from build123d import *

# Parameters (mm, degrees)
SKETCH_1_R               = 7.5
EXTRUDE_1_DEPTH          = 4
SKETCH_1_3_R             = 7.5
EXTRUDE_2_DEPTH          = 6
EXTRUDE_3_DEPTH          = 2
HOLE_WIZARD_M3_1_D       = 2.5
SKETCH_5_R               = 2.75
CUT_EXTRUDE_1_DEPTH      = 1
CUT_EXTRUDE_1_DEPTH_BACK = 4
SKETCH_6_R               = 4
CUT_EXTRUDE_2_DEPTH      = 0.75


with BuildPart() as part:
    # 草图1 → 凸台-拉伸1 (new body)
    with BuildSketch(Plane(origin=(0, 0, 0), x_dir=(1, 0, 0), z_dir=(0, 1, 0))):
        Circle(SKETCH_1_R)
        with BuildLine():
            Line((0, 3), (24.5, 3))
            ThreePointArc((24.5, 3), (27.5, 0), (24.5, -3))
            Line((24.5, -3), (0, -3))
            ThreePointArc((0, -3), (-3, 0), (0, 3))
        make_face()
    extrude(amount=EXTRUDE_1_DEPTH)

    # 草图1<3> → 凸台-拉伸2 (add)
    with BuildSketch(Plane(origin=(0, 0, 0), x_dir=(1, 0, 0), z_dir=(0, 1, 0))):
        Circle(SKETCH_1_3_R)
    extrude(amount=EXTRUDE_2_DEPTH)

    # 草图2 → 凸台-拉伸3 (add)
    with BuildSketch(Plane(origin=(0, 4, 0), x_dir=(1, 0, 0), z_dir=(0, 1, 0))):
        with BuildLine():
            Line((20, -2.5), (24, -2.5))
            ThreePointArc((24, -2.5), (26.5, 0), (24, 2.5))
            Line((24, 2.5), (20, 2.5))
            ThreePointArc((20, 2.5), (17.5, 0), (20, -2.5))
        make_face()
    extrude(amount=EXTRUDE_3_DEPTH)

    # M3 螺纹孔1 (through all)
    with Locations(Plane.XZ):
        with Locations((20, 0), (24, 0), (0, 0), (9, 0)):
            Hole(HOLE_WIZARD_M3_1_D / 2)

    # 草图5 → 切除-拉伸1 (cut, two sides)
    with BuildSketch(Plane(origin=(0, 6, 0), x_dir=(1, 0, 0), z_dir=(0, 1, 0))) as cut_extrude_1_sk:
        Circle(SKETCH_5_R)
    extrude(amount=CUT_EXTRUDE_1_DEPTH, mode=Mode.SUBTRACT)
    extrude(cut_extrude_1_sk.sketch, amount=-CUT_EXTRUDE_1_DEPTH_BACK, mode=Mode.SUBTRACT)

    # 草图6 → 切除-拉伸2 (cut)
    with BuildSketch(Plane.XZ):
        Circle(SKETCH_6_R)
    extrude(amount=-CUT_EXTRUDE_2_DEPTH, mode=Mode.SUBTRACT)


solid = part.part
Source: CAD feature listing. Evaluate the final solid. Frame: model axes, mm. A direction names the side the tool comes from. Give positions to 0.01 mm unless a question says otherwise; leave off trailing zeros. Write each loop counter-clockwise with the first axis right and the second up, starting at its lowest first coordinate (ties: lowest second). Pieces come first, ordered by that corner, then holes. Notation, with made-up numbers: (46, 25) -> (94, 25) arc R26 ccw to (94, 42) -> close; hole circle Ø1 at (68.5, 60.5). An arc over 180 degrees is marked (long way). Write item = value, one per line.
Q1. Mould query, pull axis X, two halves, no side actions, for faces 1 (the face through (-0.596, 4.028, 2.685)), 2 (the face through (6, 0, 0)), 3 (the face through (-0.867, 0.37, -3.905)), 4 (the face through (26.5, 5, 0.1)). Classes: +X half, -X half, draft (parallel to the pull), parting line (faces both ways), or undercut.
Here are the results:
face_1 = undercut
face_2 = draft
face_3 = undercut
face_4 = +X half
Q2. First-contact query: pin 1 (2 mm diameter, centred on x = 9, z = 0, fed in from -Y); pin 2 (2 mm diameter, centred on x = 21, y = 4.5, fed in from -Z); pin 3 (3.5 mm diameter, centred on x = 0, z = 0, fed in from +Y); pin 4 (2 mm diameter, centred on x = 18.5, y = 1.5, fed in from +Z). Flat tips, straight axial feed; report the tip coordinate or a pass-through.
Here are the results:
pin_1 = through
pin_2 = -3
pin_3 = 2
pin_4 = 3
Q3. Reachability of faces 5 (the face through (1, 0.75, 1)), 6 (the face through (1, 2, 1)), 7 (the face through (22, 5, 2.5)), 8 (the face through (16, 2, -3)), 9 (the face through (22, 5, -2.5)) from +Z, -Z, +X, -X, +Y, -Y: full face, straight path, thin tool, end or side. Return the list, or none.
Here are the results:
face_5 = -Y
face_6 = +Y
face_7 = +Z, +X, +Y
face_8 = -Z, +X, +Y, -Y
face_9 = -Z, +X, +Y
Q4. Cut plane B-B on y = 4.4. Return loops of the section in (x, z).
Here are the results:
outline = circle Ø15 at (0, 0); (20, -2.5) -> (24, -2.5) arc R2.5 ccw to (24, 2.5) -> (20, 2.5) arc R2.5 ccw to start; hole circle Ø5.5 at (0, 0); hole circle Ø2.5 at (20, 0); hole circle Ø2.5 at (24, 0)
Q5. Cut plane C-C on z = 0. State how many separate pieces and enclosed holes the cut face has, then the cut area to 3 significant figures.
Here are the results:
separate_pieces = 5
enclosed_holes = 0
area = 117 mm²
Q6. Line query: line 1 (Z direction, x = 0, y = 5); line 2 (Z direction, x = 24, y = 1.9); line 3 (X direction, y = 1.85, z = -0.5). Output: solid intervals per line, ascending. Write a range as from..to.
Here are the results:
line_1 = -7.5..-2.75, 2.75..7.5
line_2 = -3..-1.25, 1.25..3
line_3 = -7.48..-1.15, 1.15..7.85, 10.15..18.85, 21.15..22.85, 25.15..27.46
Q7. Cut plane A-A on x = 0. Return loops of the section in (y, z), then the cut area to 3 significant figures.
Here are the results:
outline = (0, -7.5) -> (6, -7.5) -> (6, -2.75) -> (2, -2.75) -> (2, -1.25) -> (0.75, -1.25) -> (0.75, -4) -> (0, -4) -> close; (0, 4) -> (0.75, 4) -> (0.75, 1.25) -> (2, 1.25) -> (2, 2.75) -> (6, 2.75) -> (6, 7.5) -> (0, 7.5) -> close
area = 58.9 mm²
Q8. Cut plane D-D on x = 18. Return loops of the section in (y, z), then the cut area to 3 significant figures.
Here are the results:
outline = (0, -3) -> (4, -3) -> (4, -1.5) -> (6, -1.5) -> (6, 1.5) -> (4, 1.5) -> (4, 3) -> (0, 3) -> close
area = 30.0 mm²
